```python
from build123d import *

# Parameters (mm, degrees)
EXTRUDE_1_DEPTH     = 3
SKETCH_2_R          = 1.6
SKETCH_2_R_2        = 2.6
CUT_EXTRUDE_1_DEPTH = 68.149087857
FILLET_1_R          = 10


with BuildPart() as part:
    # 草图1 → 凸台-拉伸1 (new body)
    with BuildSketch(Plane(origin=(0, 0, 0), x_dir=(1, 0, 0), z_dir=(0, 1, 0))):
        Polygon((0, -30), (0, 30), (21.715728753, 30), (60, 30), (60, -30), (21.715728753, -30), align=None)
    extrude(amount=EXTRUDE_1_DEPTH)

    # 草图2 → 切除-拉伸1 (cut, through all)
    with BuildSketch(Plane(origin=(0, 3, 0), x_dir=(1, 0, 0), z_dir=(0, 1, 0))):
        with Locations(Location((20, 7.5, 0), (0, 0, 270))):
            Circle(SKETCH_2_R)
        with Locations(Location((30, 7.5, 0), (0, 0, 270))):
            Circle(SKETCH_2_R)
        with Locations(Location((30, -7.5, 0), (0, 0, 90))):
            Circle(SKETCH_2_R)
        with Locations(Location((20, -7.5, 0), (0, 0, 90))):
            Circle(SKETCH_2_R)
        with Locations(Location((10, 20, 0), (0, 0, 270))):
            Circle(SKETCH_2_R_2)
        with Locations(Location((10, -20, 0), (0, 0, 270))):
            Circle(SKETCH_2_R_2)
        with Locations(Location((25, 20, 0), (0, 0, 270))):
            Circle(SKETCH_2_R_2)
        with Locations(Location((25, -20, 0), (0, 0, 270))):
            Circle(SKETCH_2_R_2)
        with Locations(Location((50, 17.5, 0), (0, 0, 270))):
            Circle(SKETCH_2_R_2)
        with Locations(Location((50, -17.5, 0), (0, 0, 270))):
            Circle(SKETCH_2_R_2)
    extrude(amount=-CUT_EXTRUDE_1_DEPTH, mode=Mode.SUBTRACT)

    # 圆角1
    fillet_1_edges = [part.edges().sort_by_distance(p)[0] for p in [
        (60, 1.5, -30),
        (60, 1.5, 30),
        (0, 1.5, 30),
        (0, 1.5, -30),
    ]]
    fillet(fillet_1_edges, radius=FILLET_1_R)


solid = part.part
```
Model file for the job. Use its own axes, mm. Coordinates: 2 decimals unless noted, no trailing zeros. Write each loop counter-clockwise with the first axis right and the second up, starting at its lowest first coordinate (ties: lowest second). Pieces come first, ordered by that corner, then holes. Notation, with made-up numbers: (32.5, 36) - (37.5, 36) arc R21 cw to (37.5, 43) - close; hole circle Ø2 at (43.25, 47). An arc over 180 degrees is marked (long way). One line per item, written item: value. Start each with the question number.
1. Slice it at D-D (z = 24). Write the cut outline in (x, y).
2. Flat gauge pin, fed straight in: pin 1 (3.5 mm diameter, centred on x = 20, z = -7.5, fed in from -Y). Where does the tip first touch, or does it go through?
3. Slice it at C-C (y = 2.2). Count the separate pieces of the cut face and the enclosed holes in it, plus the area to 3 significant figures.
4. Mould opens along Z. For faces 1 (the cylindrical face through (56.99, 1.52, -27.15)), 2 (the flat face through (60, 1, 0)), 3 (the cylindrical face through (31.586, 1.521, -7.708)), 4 (the cylindrical face through (56.99, 1.52, 27.15)) say: released by +Z, released by -Z, zero draft, split by the parting line, or undercut.
5. Slice it at A-A (x = 26). Write the cut outline in (y, z).
6. Slice it at B-B (z = -7.5). Write the cut outline in (x, y).
7. Probe line 1 (X direction, y = 2.25, z = 7.5); line 2 (Z direction, x = 51, y = 1.55); line 3 (Z direction, x = 50.5, y = 2.7). List the from-to ranges inside material, lowest first. Write a range as from..to.
Answers below:
1. outline: (0.83, 0) - (59.17, 0) - (59.17, 3) - (0.83, 3) - close
2. pin 1: stops at y = 0
3. separate pieces: 1
3. enclosed holes: 10
3. area: 3,350 mm^2
4. face 1: released by -Z
4. face 2: zero draft
4. face 3: undercut
4. face 4: released by +Z
5. outline: (0, -30) - (3, -30) - (3, -22.4) - (0, -22.4) - close; (0, -17.6) - (3, -17.6) - (3, 17.6) - (0, 17.6) - close; (0, 22.4) - (3, 22.4) - (3, 30) - (0, 30) - close
6. outline: (0, 0) - (18.4, 0) - (18.4, 3) - (0, 3) - close; (21.6, 0) - (28.4, 0) - (28.4, 3) - (21.6, 3) - close; (31.6, 0) - (60, 0) - (60, 3) - (31.6, 3) - close
7. line 1: x = 0..18.4, 21.6..28.4, 31.6..60
7. line 2: z = -29.95..-19.9, -15.1..15.1, 19.9..29.95
7. line 3: z = -29.99..-20.05, -14.95..14.95, 20.05..29.99
